Geometry: see drawing. Coordinates: mm, zero at the bounding-box minimum. Coordinates: 2 decimals unless noted, no trailing zeros. Loops run counter-clockwise (first coordinate to the right, second up) from the corner with the lowest first, then second, coordinate; pieces in that order, holes last. Notation, with made-up numbers: M 20,86 L 27,86 A27 cw 27,108 Z; hole C 52.5,22.5 d6. An arc over 180 degrees is marked long. One line per question, with ' | ' between items. Start each with the question number.
1. Section query D-D, the plane z = 3.5. Output: boundary loops of the cut face in (x, y), and give its area (3 significant figures).
2. Section query A-A, the plane z = 16. Output: boundary loops of the cut face in (x, y) (1 decimal), and give its area (3 significant figures).
3. Section query C-C, the plane x = 11.5. Output: boundary loops of the cut face in (y, z) (1 decimal).
4. Mould query, pull axis Y, two halves, no side actions, for the marked faces 1, 2 and 3. Classes: pulls with the +Y half, pulls with the -Y half, needs draft (parallel to the pull), parting line crosses it, or undercut.
5. Pin query (flat end, axial travel): P1, Ø4, axis at x = 16.5, z = 4.5, coming from the +Y side (1 decimal); P2, Ø5, axis at x = 28, z = 23, coming from the -Y side; P3, Ø1.5, axis at x = 15, y = 18, coming from the -Z side. Return the tip coordinate at first contact, or that it passes through.
6. Ray query, probe 1 along Y at (x, z) = (29.5, 8); probe 2 along Y at (x, z) = (13, 16); probe 3 along X at (y, z) = (18, 6). Return the intervals inside material, ascending.
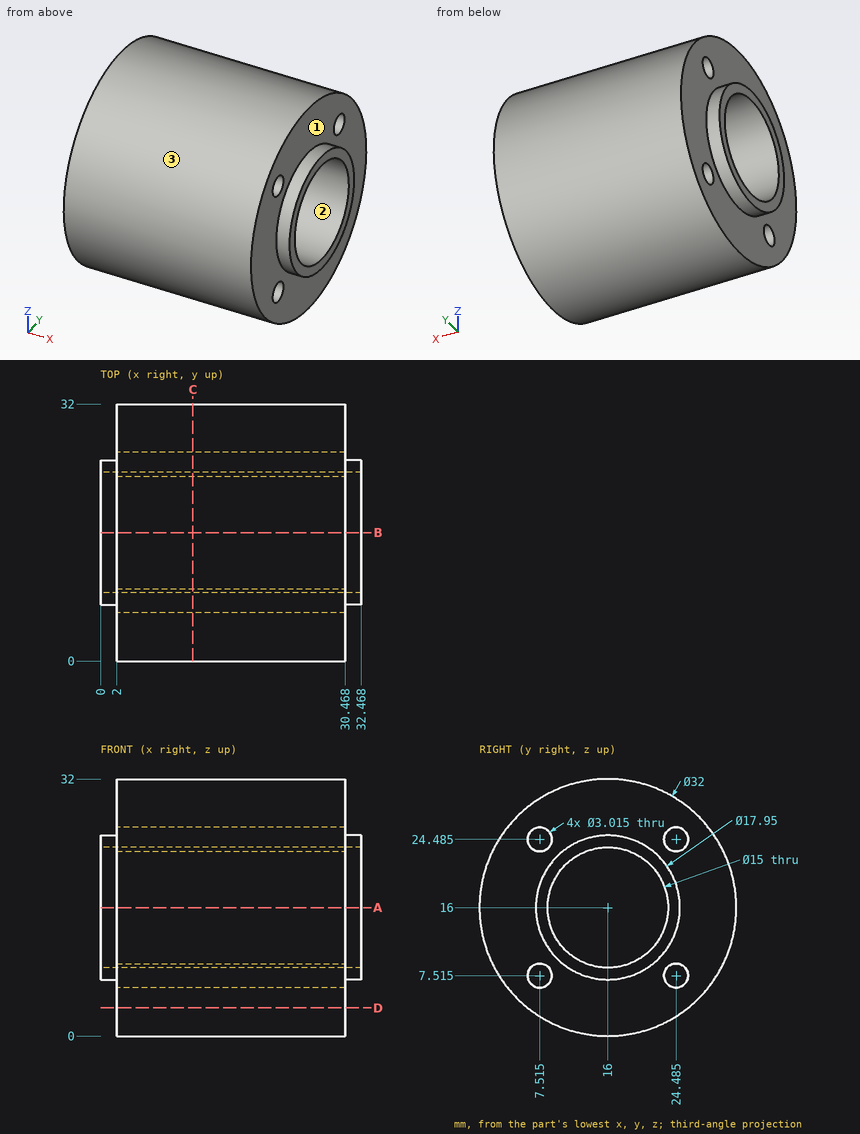
Taken from the geometry:
1) outline: M 2,6.01 L 30.47,6.01 L 30.47,25.99 L 2,25.99 Z | area: 569 mm^2
2) outline: M 0,7 L 2,7 L 2,0 L 30.5,0 L 30.5,7 L 32.5,7 L 32.5,8.5 L 0,8.5 Z; M 0,23.5 L 32.5,23.5 L 32.5,25 L 30.5,25 L 30.5,32 L 2,32 L 2,25 L 0,25 Z | area: 496 mm^2
3) outline: C 16,16 d32; hole C 7.5,7.5 d3; hole C 7.5,24.5 d3; hole C 16,16 d15; hole C 24.5,7.5 d3; hole C 24.5,24.5 d3
4) face 1: needs draft | face 2: undercut | face 3: parting line crosses it
5) P1: y = 28.9 | P2: y = 0.65 | P3: z = 0.05
6) probe 1: 2.14 to 6.09, 8.94 to 23.06, 25.91 to 29.86 | probe 2: 0 to 8.5, 23.5 to 32 | probe 3: 2 to 30.47
